Autodesk Inventor part; units mm, degrees
ref_plane "YZ Plane" through (0, 0, 0) normal (1, 0, 0) x (0, 1, 0)
ref_plane "XZ Plane" through (0, 0, 0) normal (0, 1, 0) x (-1, 0, 0)
ref_plane "XY Plane" through (0, 0, 0) normal (0, 0, 1) x (1, 0, 0)
sketch "Sketch1" plane through (0, 0, 0) normal (0, 0, 1) x (1, 0, 0)
  circle A0 centre (0, 0) radius 3.175
  line L0 (3.2079, 5.5563) -> (6.4158, 0)
  line L1 (6.4158, 0) -> (3.2079, -5.5562)
  line L2 (3.2079, -5.5562) -> (-3.2079, -5.5562)
  line L3 (-3.2079, -5.5562) -> (-6.4158, 0)
  line L4 (-6.4158, 0) -> (-3.2079, 5.5563)
  line L5 (-3.2079, 5.5563) -> (3.2079, 5.5563)
  dimension "d0" = 6.35
  dimension "d1" = 11.1125
extrude "Extrusion1" add sketch "Sketch1" against normal blind 50.8 contours A0
extrude "Extrusion2" add sketch "Sketch1" along normal blind 3.175 contours A0 | L0 L1 L2 L3 L4 L5
thread "Thread1"
chamfer "Chamfer1" distance 0.7937 angle 45 6 edges at (4.8119, 2.7781, 3.175) (0, 5.5563, 3.175) (-4.8119, 2.7781, 3.175) (-4.8119, -2.7781, 3.175) (0, -5.5562, 3.175) (4.8119, -2.7781, 3.175)
properties part number "2_bolt_.25_20"
Read the model definition and answer for the solid it produces. Units are mm, in the model's axes. A direction names the side the tool comes from. Round coordinates to 2 decimals unless told otherwise and drop trailing zeros. Write each loop counter-clockwise with the first axis right and the second up, starting at its lowest first coordinate (ties: lowest second). Pieces come first, ordered by that corner, then holes.
1. Straight lines are drawn through the part: L1, parallel to X at y = -0.25, z = -41.5; L2, parallel to Z at x = 2, y = 2.5 (3 decimals). For each, find the intervals that lie inside material, in ascending order.
2. The part is cut by section C-C, the plane z = -3. Determine the outline of the cut face in (x, y) (3 decimals), then the cut area to 3 significant figures.
3. The part is cut by section B-B, the plane y = 1.5. Determine the outline of the cut face in (x, z) (3 decimals).
4. Which of the six approach directions +Z, -Z, +X, -X, +Y, -Y give full straight-line access (tool end or side, diameter ignored) to faces 1 (the face through (-0.69, -3.1, -25.04)), 2 (the face through (4.44, -2.62, 2.78))?
5. The part is cut by section A-A, the plane x = 0. Determine the outline of the cut face in (y, z) (1 decimal).
6. The part is cut by section D-D, the plane x = 4.5. Determine the outline of the cut face in (y, z) (3 decimals).
7. Given pin 1 Ø4 at (x, z) = (-1.5, -18.5) entering from -Y (3 decimals); pin 2 Ø1.5 at (x, z) = (0, -25) entering from +Y (3 decimals); pin 3 Ø4 at (x, y) = (-4, 0) entering from -Z; pin 4 Ø1.5 at (y, z) = (0.5, -19.5) entering from +X (3 decimals), each flat-ended and moving along its own axis, determine where each tip first touches the part or whether it passes through.
Values:
1. L1: x = -3.17 to 3.17
1. L2: z = 0 to 3.175
2. outline: circle Ø6.35 at (0, 0)
2. area: 31.7 mm2
3. outline: (-5.55, 0) - (-2.798, 0) - (-2.798, -50.8) - (2.798, -50.8) - (2.798, 0) - (5.55, 0) - (5.55, 2.381) - (4.633, 3.175) - (-4.633, 3.175) - (-5.55, 2.381) - close
4. face 1: -Z
4. face 2: +Z, +X, -Y
5. outline: (-5.6, 0) - (-3.2, 0) - (-3.2, -50.8) - (3.2, -50.8) - (3.2, 0) - (5.6, 0) - (5.6, 2.4) - (4.8, 3.2) - (-4.8, 3.2) - (-5.6, 2.4) - close
6. outline: (-3.318, 0) - (3.318, 0) - (3.318, 2.381) - (1.731, 3.175) - (-1.731, 3.175) - (-3.318, 2.381) - close
7. pin 1: stops at y = -3.175
7. pin 2: stops at y = 3.175
7. pin 3: stops at z = -50.8
7. pin 4: stops at x = 3.175
